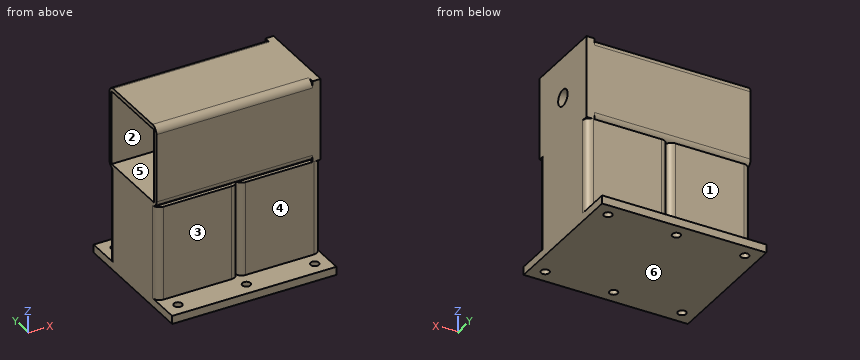
```python
from build123d import *

# Parameters (mm, degrees)
F0_W     = 54
F0_H     = 54
F1_DEPTH = 69
F2_R     = 3
F2_W     = 54
F2_H     = 54
F3_DEPTH = 6
F4_W     = 54
F4_H     = 54
F5_DEPTH = 120
F6_W     = 60
F6_H     = 60
F6_R     = 6
F7_DEPTH = 6


with BuildPart() as f1:
    # F0 (on Top) → F1 (new body)
    with BuildSketch(Plane.XY):
        with BuildLine():
            ThreePointArc((-5.85040465, -3.5986092687), (-9.3859385559, -5.0630753627), (-10.85040465, -8.5986092687))
            Line((-10.85040465, -8.5986092687), (-10.85040465, -58.5986092687))
            ThreePointArc((-10.85040465, -58.5986092687), (-9.3859385559, -62.1341431746), (-5.85040465, -63.5986092687))
            Line((-5.85040465, -63.5986092687), (44.14959535, -63.5986092687))
            ThreePointArc((44.14959535, -63.5986092687), (47.685129256, -62.1341431746), (49.14959535, -58.5986092687))
            Line((49.14959535, -58.5986092687), (49.14959535, -8.5986092687))
            ThreePointArc((49.14959535, -8.5986092687), (47.685129256, -5.0630753627), (44.14959535, -3.5986092687))
            Line((44.14959535, -3.5986092687), (-5.85040465, -3.5986092687))
        make_face()
        with Locations((19.14959535, -33.5986092687)):
            Rectangle(F0_W, F0_H, mode=Mode.SUBTRACT)
        with BuildLine():
            ThreePointArc((54.14959535, -3.5986092687), (50.6140614441, -5.0630753627), (49.14959535, -8.5986092687))
            Line((49.14959535, -8.5986092687), (49.14959535, -58.5986092687))
            ThreePointArc((49.14959535, -58.5986092687), (50.6140614441, -62.1341431746), (54.14959535, -63.5986092687))
            Line((54.14959535, -63.5986092687), (104.14959535, -63.5986092687))
            ThreePointArc((104.14959535, -63.5986092687), (107.685129256, -62.1341431746), (109.14959535, -58.5986092687))
            Line((109.14959535, -58.5986092687), (109.14959535, -8.5986092687))
            ThreePointArc((109.14959535, -8.5986092687), (107.685129256, -5.0630753627), (104.14959535, -3.5986092687))
            Line((104.14959535, -3.5986092687), (54.14959535, -3.5986092687))
        make_face()
        with Locations((79.14959535, -33.5986092687)):
            Rectangle(F0_W, F0_H, mode=Mode.SUBTRACT)
    extrude(amount=F1_DEPTH)

    # F2 (on face) → F3 (join)
    with BuildSketch(Plane(origin=(0, 0, 0), x_dir=(1, 0, 0), z_dir=(0, 0, -1))):
        with BuildLine():
            Line((-10.85040465, -16.4013907313), (109.14959535, -16.4013907313))
            Line((109.14959535, -16.4013907313), (109.14959535, 8.5986092687))
            ThreePointArc((109.14959535, 8.5986092687), (107.685129256, 5.0630753627), (104.14959535, 3.5986092687))
            Line((104.14959535, 3.5986092687), (54.14959535, 3.5986092687))
            ThreePointArc((54.14959535, 3.5986092687), (50.6140614441, 5.0630753627), (49.14959535, 8.5986092687))
            ThreePointArc((49.14959535, 8.5986092687), (47.685129256, 5.0630753627), (44.14959535, 3.5986092687))
            Line((44.14959535, 3.5986092687), (-5.85040465, 3.5986092687))
            ThreePointArc((-5.85040465, 3.5986092687), (-9.3859385559, 5.0630753627), (-10.85040465, 8.5986092687))
            Line((-10.85040465, 8.5986092687), (-10.85040465, -16.4013907313))
        make_face()
        with Locations((-0.85040465, -6.4013907313)):
            Circle(F2_R, mode=Mode.SUBTRACT)
        with Locations((49.14959535, -6.4013907313)):
            Circle(F2_R, mode=Mode.SUBTRACT)
        with Locations((99.14959535, -6.4013907313)):
            Circle(F2_R, mode=Mode.SUBTRACT)
        with BuildLine():
            ThreePointArc((104.14959535, 63.5986092687), (107.685129256, 62.1341431746), (109.14959535, 58.5986092687))
            Line((109.14959535, 58.5986092687), (109.14959535, 83.5986092687))
            Line((109.14959535, 83.5986092687), (-10.85040465, 83.5986092687))
            Line((-10.85040465, 83.5986092687), (-10.85040465, 58.5986092687))
            ThreePointArc((-10.85040465, 58.5986092687), (-9.3859385559, 62.1341431746), (-5.85040465, 63.5986092687))
            Line((-5.85040465, 63.5986092687), (44.14959535, 63.5986092687))
            ThreePointArc((44.14959535, 63.5986092687), (47.685129256, 62.1341431746), (49.14959535, 58.5986092687))
            ThreePointArc((49.14959535, 58.5986092687), (50.6140614441, 62.1341431746), (54.14959535, 63.5986092687))
            Line((54.14959535, 63.5986092687), (104.14959535, 63.5986092687))
        make_face()
        with Locations((-0.85040465, 73.5986092687)):
            Circle(F2_R, mode=Mode.SUBTRACT)
        with Locations((49.14959535, 73.5986092687)):
            Circle(F2_R, mode=Mode.SUBTRACT)
        with Locations((99.14959535, 73.5986092687)):
            Circle(F2_R, mode=Mode.SUBTRACT)
        with BuildLine():
            ThreePointArc((104.14959535, 3.5986092687), (107.685129256, 5.0630753627), (109.14959535, 8.5986092687))
            Line((109.14959535, 8.5986092687), (109.14959535, 58.5986092687))
            ThreePointArc((109.14959535, 58.5986092687), (107.685129256, 62.1341431746), (104.14959535, 63.5986092687))
            Line((104.14959535, 63.5986092687), (54.14959535, 63.5986092687))
            ThreePointArc((54.14959535, 63.5986092687), (50.6140614441, 62.1341431746), (49.14959535, 58.5986092687))
            ThreePointArc((49.14959535, 58.5986092687), (47.685129256, 62.1341431746), (44.14959535, 63.5986092687))
            Line((44.14959535, 63.5986092687), (-5.85040465, 63.5986092687))
            ThreePointArc((-5.85040465, 63.5986092687), (-9.3859385559, 62.1341431746), (-10.85040465, 58.5986092687))
            Line((-10.85040465, 58.5986092687), (-10.85040465, 8.5986092687))
            ThreePointArc((-10.85040465, 8.5986092687), (-9.3859385559, 5.0630753627), (-5.85040465, 3.5986092687))
            Line((-5.85040465, 3.5986092687), (44.14959535, 3.5986092687))
            ThreePointArc((44.14959535, 3.5986092687), (47.685129256, 5.0630753627), (49.14959535, 8.5986092687))
            ThreePointArc((49.14959535, 8.5986092687), (50.6140614441, 5.0630753627), (54.14959535, 3.5986092687))
            Line((54.14959535, 3.5986092687), (104.14959535, 3.5986092687))
        make_face()
        with Locations((19.14959535, 33.5986092687)):
            Rectangle(F2_W, F2_H, mode=Mode.SUBTRACT)
        with Locations((79.14959535, 33.5986092687)):
            Rectangle(F2_W, F2_H, mode=Mode.SUBTRACT)
        with Locations((19.14959535, 33.5986092687)):
            Rectangle(F2_W, F2_H)
        with Locations((79.14959535, 33.5986092687)):
            Rectangle(F2_W, F2_H)
    extrude(amount=F3_DEPTH)

    # F4 (on face) → F5 (join, through all)
    with BuildSketch(Plane.YZ.offset(109.14959535)):
        with BuildLine():
            ThreePointArc((-3.5986092687, 124), (-5.0630753627, 127.5355339059), (-8.5986092687, 129))
            Line((-8.5986092687, 129), (-58.5986092687, 129))
            ThreePointArc((-58.5986092687, 129), (-62.1341431746, 127.5355339059), (-63.5986092687, 124))
            Line((-63.5986092687, 124), (-63.5986092687, 74))
            ThreePointArc((-63.5986092687, 74), (-62.1341431746, 70.4644660941), (-58.5986092687, 69))
            Line((-58.5986092687, 69), (-8.5986092687, 69))
            ThreePointArc((-8.5986092687, 69), (-5.0630753627, 70.4644660941), (-3.5986092687, 74))
            Line((-3.5986092687, 74), (-3.5986092687, 124))
        make_face()
        with Locations((-33.5986092687, 99)):
            Rectangle(F4_W, F4_H, mode=Mode.SUBTRACT)
    extrude(amount=-F5_DEPTH)

    # F6 (on face) → F7 (join)
    with BuildSketch(Plane.YZ.offset(109.14959535)):
        with Locations((-33.5986092687, 99)):
            Rectangle(F6_W, F6_H)
        with Locations((-33.5986092687, 99)):
            Circle(F6_R, mode=Mode.SUBTRACT)
    extrude(amount=-F7_DEPTH)


solid = f1.part
```
The model under review builds one solid part; all positions refer to its coordinate system, in mm. Face numbers are marked on the shaded views. A direction names the side the tool comes from. Coordinates: 2 decimals unless noted, no trailing zeros. Write each loop counter-clockwise with the first axis right and the second up, starting at its lowest first coordinate (ties: lowest second). Pieces come first, ordered by that corner, then holes.
1) We need section A-A on x = 42. State the section outline as (y, z) points, then the cut area to 3 significant figures.
2) We need section D-D on y = -41.5. State the section outline as (x, z) points.
3) To check wall thickness, follow probe 1 along Z at (x, y) = (72, -25.5); probe 2 along X at (y, z) = (-43, 30.5); probe 3 along Y at (x, z) = (66, 48). State the ranges of each line that lie inside material, in increasing order.
4) We need section C-C on z = 46. State the section outline as (x, y) points, then the cut area to 3 significant figures.
5) Clearance check with flat-ended pins moving along their axes: pin 1 Ø5 at (x, y) = (99.15, -73.6) entering from +Z; pin 2 Ø6 at (x, z) = (68, 43) entering from -Y; pin 3 Ø2 at (y, z) = (-5.5, 22) entering from +X; pin 4 Ø20 at (x, y) = (19.5, -71.5) entering from +Z. State where each tip first meets the part, or that it passes through.
6) The part is to be moulded in two halves that separate along Z. For the marked faces 4, 5 and 6, say which applies: pulls with the +Z half, pulls with the -Z half, needs draft (parallel to the pull), parting line crosses it, or undercut.
7) Machinability: for the marked faces 1, 2 and 3, which of the approach directions +Z, -Z, +X, -X, +Y, -Y give a long, thin tool a straight path to every point of the face, cutting with its end or side? Answer none if there is none.
8) We need section B-B on z = 99. State the section outline as (x, y) points, then the cut area to 3 significant figures.
Answer list:
1. outline: (-83.6, -6) - (16.4, -6) - (16.4, 0) - (-3.6, 0) - (-3.6, 69) - (-6.6, 69) - (-6.6, 0) - (-60.6, 0) - (-60.6, 69) - (-63.6, 69) - (-63.6, 0) - (-83.6, 0) - close; (-63.6, 74) arc R5 ccw to (-58.6, 69) - (-8.6, 69) arc R5 ccw to (-3.6, 74) - (-3.6, 124) arc R5 ccw to (-8.6, 129) - (-58.6, 129) arc R5 ccw to (-63.6, 124) - close; hole (-60.6, 72) - (-6.6, 72) - (-6.6, 126) - (-60.6, 126) - close
1. area: 1,680 mm2
2. outline: (-10.85, -6) - (109.15, -6) - (109.15, 129) - (-10.85, 129) - (-10.85, 126) - (103.15, 126) - (103.15, 72) - (-10.85, 72) - close; hole (-7.85, 0) - (46.15, 0) - (46.15, 69) - (-7.85, 69) - close; hole (52.15, 0) - (106.15, 0) - (106.15, 69) - (52.15, 69) - close
3. probe 1: z = -6 to 0, 69 to 72, 126 to 129
3. probe 2: x = -10.85 to -7.85, 46.15 to 52.15, 106.15 to 109.15
3. probe 3: y = -63.6 to -60.6, -6.6 to -3.6
4. outline: (-10.85, -58.6) arc R5 ccw to (-5.85, -63.6) - (44.15, -63.6) arc R5 ccw to (49.15, -58.6) arc R5 ccw to (54.15, -63.6) - (104.15, -63.6) arc R5 ccw to (109.15, -58.6) - (109.15, -8.6) arc R5 ccw to (104.15, -3.6) - (54.15, -3.6) arc R5 ccw to (49.15, -8.6) arc R5 ccw to (44.15, -3.6) - (-5.85, -3.6) arc R5 ccw to (-10.85, -8.6) - close; hole (-7.85, -60.6) - (46.15, -60.6) - (46.15, -6.6) - (-7.85, -6.6) - close; hole (52.15, -60.6) - (106.15, -60.6) - (106.15, -6.6) - (52.15, -6.6) - close
4. area: 1,330 mm2
5. pin 1: passes through
5. pin 2: stops at y = -63.6
5. pin 3: stops at x = 108.69
5. pin 4: stops at z = 128.07
6. face 4: needs draft
6. face 5: undercut
6. face 6: pulls with the -Z half
7. face 1: +Z, +X, -X, +Y
7. face 2: -X
7. face 3: +Z, +X, -X, -Y
8. outline: (-10.85, -63.6) - (109.15, -63.6) - (109.15, -39.6) - (103.15, -39.6) - (103.15, -60.6) - (-10.85, -60.6) - close; (-10.85, -6.6) - (103.15, -6.6) - (103.15, -27.6) - (109.15, -27.6) - (109.15, -3.6) - (-10.85, -3.6) - close
8. area: 972 mm2
